Part model, mm, in its own coordinate system. A direction names the side the tool comes from. Give positions to 0.01 mm unless a question says otherwise; leave off trailing zeros. Loops run counter-clockwise (first coordinate to the right, second up) from the corner with the lowest first, then second, coordinate; pieces in that order, holes last. Notation, with made-up numbers: (78.5, 16.25) -> (102.5, 16.25) arc R17 ccw to (102.5, 44.25) -> close; hole circle Ø8 at (7.5, 80). An arc over 180 degrees is marked (long way). Write item = value, one per line.
from build123d import *

# Parameters (mm, degrees)
F2_DEPTH  = 20
F3_W      = 217
F3_H      = 242
F3_W_2    = 167
F3_H_2    = 192
F4_DEPTH  = 240
F5_W      = 48
F5_H      = 72
F6_DEPTH  = 250
F7_W      = 79
F7_H      = 85
F8_DEPTH  = 25
F10_DEPTH = 25
F11_DEPTH = 25
F12_DEPTH = 20


with BuildPart() as f2:
    # F1 (on face) → F2 (new body)
    with BuildSketch(Plane.XY):
        Polygon((-497, -215), (-497, -231), (-497, -293), (-497, -407), (-330, -407), (-330, -287), (-330, -215), align=None)
    extrude(amount=F2_DEPTH)

    # F3 (on face) → F4 (join)
    with BuildSketch(Plane.XY):
        with Locations((-413.5, -311)):
            Rectangle(F3_W, F3_H)
        with Locations((-413.5, -311)):
            Rectangle(F3_W_2, F3_H_2, mode=Mode.SUBTRACT)
    extrude(amount=F4_DEPTH)

    # F5 (on face) → F6 (cut)
    with BuildSketch(Plane.XY.offset(20)):
        with Locations((-306, -251)):
            Rectangle(F5_W, F5_H)
    extrude(amount=F6_DEPTH, mode=Mode.SUBTRACT)

    # F7 (on face) → F8 (cut)
    with BuildSketch(Plane.YZ.offset(-497)):
        with Locations((-309.5, 177.5)):
            Rectangle(F7_W, F7_H)
    extrude(amount=-F8_DEPTH, mode=Mode.SUBTRACT)

    # F9 (on face) → F10 (join, through all)
    with BuildSketch(Plane.YZ.offset(-497)):
        Polygon((-270, 135), (-270, 220), (-290, 220), (-290, 155), (-349, 155), (-349, 135), align=None)
    extrude(amount=-F10_DEPTH)

    # F11 (cut): a face of the model
    f11_faces = [f2.faces().sort_by_distance(p)[0] for p in [
        (-408.3972360028, -307.8107725018, 20),
    ]]
    extrude(f11_faces, amount=-F11_DEPTH, mode=Mode.SUBTRACT)

    # F12 (cut): a face of the model
    f12_faces = [f2.faces().sort_by_distance(p)[0] for p in [
        (-308.2504307407, -202.5, 0),
    ]]
    extrude(f12_faces, amount=-F12_DEPTH, mode=Mode.SUBTRACT)


solid = f2.part
1) Pull direction Z, two halves, no side cores. Call faces 1 (the face through (-497, -312, 132)), 2 (the face through (-509, -319, 155)), 3 (the face through (-502, -310, 20)): pulls with the +Z half, pulls with the -Z half, needs draft (parallel to the pull), parting line crosses it, or undercut.
Resolved:
face_1 = needs draft
face_2 = undercut
face_3 = pulls with the -Z half
2) Drop a flat-ended pin along its axis: P1, Ø10, axis at y = -299, z = 204.5, coming from the -X side. Give the stop position or say it passes through.
Resolved:
P1 = -330
3) Which spindle directions (+Z, -Z, +X, -X, +Y, -Y) get a long thin tool onto all of the face, cutting with end or side? Do faces 4 (the face through (-509, -349, 187)), 5 (the face through (-415, -407, 128)), 6 (the face through (-502, -310, 240)), 7 (the face through (-318, -287, 128)). Say none if no direction does.
Resolved:
face_4 = -X
face_5 = +Z, -Z
face_6 = +Z, +X, -X, +Y, -Y
face_7 = +Z, -Z, +X
4) Slice it at C-C, the plane z = 186.5. List the corners of the cut face in (x, y), and give its area (3 significant figures).
Resolved:
outline = (-522, -432) -> (-305, -432) -> (-305, -287) -> (-330, -287) -> (-330, -407) -> (-497, -407) -> (-497, -349) -> (-522, -349) -> close; (-522, -290) -> (-497, -290) -> (-497, -215) -> (-305, -215) -> (-305, -190) -> (-522, -190) -> close
area = 17,200 mm²
5) Slice it at A-A, the plane x = -324.5. List the corners of the cut face in (y, z).
Resolved:
outline = (-432, 20) -> (-287, 20) -> (-287, 240) -> (-432, 240) -> close; (-215, 20) -> (-190, 20) -> (-190, 240) -> (-215, 240) -> close
6) Drill centre lines: line 1 along Y through (x, z) = (-421.5, 46.5); line 2 along X through (y, z) = (-350, 52.5); line 3 along Z through (x, y) = (-498, -291.5). Where is each one in solid material? Low to high. Write a range as [from, to].
Resolved:
line_1 = [-432, -407], [-215, -190]
line_2 = [-522, -497], [-330, -305]
line_3 = [20, 155], [220, 240]
7) Slice it at B-B, the plane y = -354. List the corners of the cut face in (x, z), and give its area (3 significant figures).
Resolved:
outline = (-522, 20) -> (-497, 20) -> (-497, 240) -> (-522, 240) -> close; (-330, 20) -> (-305, 20) -> (-305, 240) -> (-330, 240) -> close
area = 11,000 mm²
8) Slice it at D-D, the plane z = 65. List the corners of the cut face in (x, y), and give its area (4 significant figures).
Resolved:
outline = (-522, -432) -> (-305, -432) -> (-305, -287) -> (-330, -287) -> (-330, -407) -> (-497, -407) -> (-497, -215) -> (-305, -215) -> (-305, -190) -> (-522, -190) -> close
area = 18,650 mm²
